Read the model definition and answer for the solid it produces. Units are mm, in the model's axes. Coordinates: 2 decimals unless noted, no trailing zeros. Write each loop counter-clockwise with the first axis right and the second up, starting at its lowest first coordinate (ties: lowest second). Pieces come first, ordered by that corner, then holes.
1) The part is cut by section A-A (y = 33.5). Determine the outline of the cut face in (x, z) (3 decimals).
2) Each of these flat-tipped pins is pushed along its axis until it touches: pin 1 Ø1 at (y, z) = (20, -544.5) entering from +X; pin 2 Ø1.6 at (x, z) = (2, -502.5) entering from -Y. Where does it stop, or does it pass through?
3) The part is cut by section B-B (x = 1.2). Give the number of separate pieces and of enclosed holes in the cut face, then the cut area to 3 significant figures.
4) Find the intervals of material crossed by line 1 (Z direction, x = 0.2, y = 31) (3 decimals); line 2 (Y direction, x = 1.85, z = -95.25); line 3 (Y direction, x = 2.1, z = -381), in increasing order.
from build123d import *

# Parameters (mm, degrees)
SKETCH2_W                    = 758.825
SKETCH2_H                    = 100.0125
BOSS_EXTRUDE1_DEPTH          = 3.175
F_10_0_1935_DIAMETER_HOLE2_D = 4.9149
SKETCH7_W                    = 38.1
SKETCH7_H                    = 44.45
CUT_EXTRUDE3_DEPTH           = 254


with BuildPart() as part:
    # Sketch2 → Boss-Extrude1 (new body)
    with BuildSketch(Plane(origin=(0, 0, 0), x_dir=(0, 0, -1), z_dir=(1, 0, 0))):
        with Locations((379.4125, 50.00625)):
            Rectangle(SKETCH2_W, SKETCH2_H)
    extrude(amount=BOSS_EXTRUDE1_DEPTH)

    # #10 (0.1935) Diameter Hole2 (through all)
    with Locations(Plane(origin=(3.175, 0, 0), x_dir=(0, 0, -1), z_dir=(1, 0, 0))):
        with Locations((19.05, 84.1375), (379.4125, 84.1375), (739.775, 84.1375), (95.25, 19.05), (381, 19.05), (542.9885, 19.05), (714.375, 19.05)):
            Hole(F_10_0_1935_DIAMETER_HOLE2_D / 2)

    # Sketch7 → Cut-Extrude3 (cut)
    with BuildSketch(Plane(origin=(3.175, 0, 0), x_dir=(0, 0, -1), z_dir=(1, 0, 0))):
        with Locations((511.175, 22.225)):
            Rectangle(SKETCH7_W, SKETCH7_H)
    extrude(amount=-CUT_EXTRUDE3_DEPTH, mode=Mode.SUBTRACT)


solid = part.part
Reported:
1. outline: (0, -758.825) - (3.175, -758.825) - (3.175, -530.225) - (0, -530.225) - close; (0, -492.125) - (3.175, -492.125) - (3.175, 0) - (0, 0) - close
2. pin 1: passes through
2. pin 2: stops at y = 44.45
3. separate pieces: 1
3. enclosed holes: 7
3. area: 74,100 mm2
4. line 1: z = -758.825 to -530.225, -492.125 to 0
4. line 2: y = 0 to 16.59, 21.51 to 100.01
4. line 3: y = 0 to 16.59, 21.51 to 82.26, 86.01 to 100.01
